```python
from build123d import *

# Parameters (mm, degrees)
EXTRUDE_THIN1_DEPTH = 5


with BuildPart() as part:
    # Sketch2 → Extrude-Thin1 (new body)
    with BuildSketch(Plane.XY):
        with BuildLine():
            Line((31.737189524, 49.429256179), (18.452031438, 5.005116936))
            ThreePointArc((18.452031438, 5.005116936), (2.455857834, -3.849946484), (-6.741752404, 11.951752286))
            Line((-6.741752404, 11.951752286), (18.457702948, 111.680824527))
            ThreePointArc((18.457702948, 111.680824527), (52.139902973, 127.701671453), (61.588984186, 91.620194226))
            Line((61.588984186, 91.620194226), (32.759580087, 51.509058335))
            ThreePointArc((32.759580087, 51.509058335), (32.16171614, 50.511761899), (31.737189524, 49.429256179))
        make_face()
        with BuildLine():
            Line((26.946810916, 50.86183176), (13.66165283, 6.437692517))
            ThreePointArc((13.66165283, 6.437692517), (3.784902946, 0.97018205), (-1.894111179, 10.726854512))
            Line((-1.894111179, 10.726854512), (23.305344172, 110.455926753))
            ThreePointArc((23.305344172, 110.455926753), (50.031286447, 123.168048581), (57.528884552, 94.538342776))
            Line((57.528884552, 94.538342776), (28.699480452, 54.427206885))
            ThreePointArc((28.699480452, 54.427206885), (27.674570829, 52.717555851), (26.946810916, 50.86183176))
        make_face(mode=Mode.SUBTRACT)
    extrude(amount=EXTRUDE_THIN1_DEPTH)


solid = part.part
```
Work out the finished part from the listing and answer in its coordinate system (mm). A direction names the side the tool comes from. Give positions to 0.01 mm unless a question says otherwise; leave off trailing zeros. Loops run counter-clockwise (first coordinate to the right, second up) from the corner with the lowest first, then second, coordinate; pieces in that order, holes last. Notation, with made-up numbers: (-14, -2) -> (33, -2) arc R13 ccw to (33, 19) -> close; hole circle Ø5 at (80.25, -31.75). An arc over 180 degrees is marked (long way). Write item = value, one per line. Start each with the question number.
(1) Find the intervals of material crossed by probe 1 along X at (y, z) = (55, 1.95); probe 2 along X at (y, z) = (49, 1.9); probe 3 along Y at (x, z) = (52, 1.7), in increasing order. Write a range as from..to.
(2) Find section A-A on z = 1.6. Give the vertices of the cut face in (x, y).
(3) Which of the six approach directions +Z, -Z, +X, -X, +Y, -Y give full straight-line access (tool end or side, diameter ignored) to faces 5 (the cylindrical face through (27.687, 52.743, 2.465)), 6 (the flat face through (47.38, 71.85, 2.46))?
(4) Find section B-B on x = 1. Give the vertices of the cut face in (y, z), and give its area (3 significant figures).
(5) Find section C-C on y = 76.5. Give the vertices of the cut face in (x, z), and give its area (3 significant figures).
(6) Given pin 1 Ø1 at (y, z) = (51, 3.5) entering from +X; pin 2 Ø1.5 at (x, z) = (21.5, 2.5) entering from +Y; pin 3 Ø1 at (x, z) = (42.5, 1.5) entering from -Y, each flat-ended and moving along its own axis, determine where each tip first touches the part or whether it passes through.
(7) The mould has two halves that part along X. Classify faces 1 (the flat face through (43.316, 74.764, 2.465)), 2 (the cylindrical face through (51.596, 127.946, 2.465)), 3 (the flat face through (32, 58, 0)), 4 (the flat face through (5.68, 61.12, 2.46)): +X half, -X half, draft (parallel to the pull), parting line (faces both ways), or undercut.
From the geometry:
q1.probe_1 = 4.14..9.29, 29.11..35.27
q1.probe_2 = 2.62..7.78, 26.39..31.61
q1.probe_3 = 78.28..86.85, 122.11..127.77
q2.outline = (-6.74, 11.95) arc R13.07 ccw to (18.45, 5.01) -> (31.74, 49.43) arc R7 cw to (32.76, 51.51) -> (61.59, 91.62) arc R24.21 ccw (long way) to (18.46, 111.68) -> close; hole (-1.89, 10.73) arc R8.07 ccw to (13.66, 6.44) -> (26.95, 50.86) arc R12 cw to (28.7, 54.43) -> (57.53, 94.54) arc R19.21 ccw (long way) to (23.31, 110.46) -> close
q3.face_5 = +Z, -Z
q3.face_6 = +Z, -Z, +X, -Y
q4.outline = (-3.35, 0) -> (2.36, 0) -> (2.36, 5) -> (-3.35, 5) -> close; (22.18, 0) -> (42.59, 0) -> (42.59, 5) -> (22.18, 5) -> close
q4.area = 131 mm^2
q5.outline = (9.57, 0) -> (14.73, 0) -> (14.73, 5) -> (9.57, 5) -> close; (44.56, 0) -> (50.72, 0) -> (50.72, 5) -> (44.56, 5) -> close
q5.area = 56.6 mm^2
q6.pin_1 = 32.75
q6.pin_2 = 119.85
q6.pin_3 = 64.37
q7.face_1 = undercut
q7.face_2 = parting line
q7.face_3 = draft
q7.face_4 = -X half
